Build history of the part. All positions in model axes, mm. A direction names the side the tool comes from. Round coordinates to 2 decimals unless told otherwise and drop trailing zeros. Write each loop counter-clockwise with the first axis right and the second up, starting at its lowest first coordinate (ties: lowest second). Pieces come first, ordered by that corner, then holes. Notation, with made-up numbers: (-9, 50.25) - (33, 50.25) arc R22 cw to (33, 79.25) - close; hole circle Ø3 at (37, 3.5). An arc over 180 degrees is marked (long way). Answer as a JSON object with one key per item and string values. Group by question number.
Item 1: Probe line 1 (Y direction, x = 14, z = -1.75); line 2 (Y direction, x = 37, z = -0.25). List the from-to ranges inside material, lowest first. Write a range as from..to.
Item 2: Slice it at A-A, the plane z = 0. List the corners of the cut face in (x, y) (3 decimals), then the cut area to 3 significant figures.
Item 3: Slice it at B-B, the plane y = 0. List the corners of the cut face in (x, z) (3 decimals).
Item 4: Two-plate mould, pull along Y, no slides. Class faces 3 (the cylindrical face through (24.46, -2.861, 9.085)), 4 (the flat face through (50.8, 0, 0)), 5 (the flat face through (3, 1.702, 0)): +Y half, -Y half, draft (parallel to the pull), parting line (faces both ways), or undercut.
Item 5: Slice it at D-D, the plane x = 40.5. List the corners of the cut face in (y, z) (3 decimals), then the cut area to 3 significant figures.
Item 6: Which spindle directions (+Z, -Z, +X, -X, +Y, -Y) get a long thin tool onto all of the face, cutting with end or side? Do faces 1 (the flat face through (4.902, 0, 0)), 2 (the conical face through (50.56, 5.28, 2.75)). Say none if no direction does.
Item 7: Flat gauge pins, fed straight in: pin 1 (2 mm diameter, centred on x = 37, y = 6, fed in from +Z); pin 2 (5.5 mm diameter, centred on x = 1.5, z = 2.5, fed in from +Y) (3 decimals); pin 3 (10 mm diameter, centred on x = 26, y = 6, fed in from +Z); pin 4 (1.5 mm diameter, centred on x = 33.5, y = -6.5, fed in from +Z). Where does each tip first touch, or does it go through?
Item 8: Slice it at C-C, the plane x = 3.5. List the corners of the cut face in (y, z) (3 decimals), then the cut area to 3 significant figures.
from build123d import *

# Parameters (mm, degrees)
SKETCH2_W  = 19.05
SKETCH2_H  = 3.4036
SLOT_DEPTH = 4.9022


with BuildPart() as part:
    # BodySke → BaseBody (revolve)
    with BuildSketch(Plane.XY, mode=Mode.PRIVATE) as basebody_sk:
        with BuildLine():
            Line((50.8, 0), (50.8, 5.715))
            Line((50.8, 5.715), (46.99, 9.525))
            Line((46.99, 9.525), (2.552216058, 9.525))
            ThreePointArc((2.552216058, 9.525), (0.649113009, 4.930502809), (0, 0))
            Line((0, 0), (50.8, 0))
        make_face()
    revolve(basebody_sk.sketch.rotate(Axis((-12.7, 0, 0), (1, 0, 0)), 90), axis=Axis((-12.7, 0, 0), (1, 0, 0)))

    # Sketch2 → Slot (cut)
    with BuildSketch(Plane(origin=(0, 0, 0), x_dir=(0, 0, -1), z_dir=(1, 0, 0))):
        Rectangle(SKETCH2_W, SKETCH2_H)
    extrude(amount=SLOT_DEPTH, mode=Mode.SUBTRACT)


solid = part.part
Geometry says:
{
 "1": {"line 1": "y = -9.36..9.36", "line 2": "y = -9.52..9.52"},
 "2": {"outline": "(0.076, -1.702) arc R19.05 ccw to (2.552, -9.525) - (46.99, -9.525) - (50.8, -5.715) - (50.8, 5.715) - (46.99, 9.525) - (2.552, 9.525) arc R19.05 ccw to (0.076, 1.702) - (4.902, 1.702) - (4.902, -1.702) - close", "area": "921 mm^2"},
 "3": {"outline": "(4.902, -9.525) - (46.99, -9.525) - (50.8, -5.715) - (50.8, 5.715) - (46.99, 9.525) - (4.902, 9.525) - close"},
 "4": {"face 3": "parting line", "face 4": "draft", "face 5": "undercut"},
 "5": {"outline": "circle Ø19.05 at (0, 0)", "area": "285 mm^2"},
 "6": {"face 1": "+Z, -Z, -X", "face 2": "+X"},
 "7": {"pin 1": "stops at z = 8.11", "pin 2": "stops at y = 9.525", "pin 3": "stops at z = 9.47", "pin 4": "stops at z = 7.59"},
 "8": {"outline": "(-1.702, -9.372) - (-1.702, 9.372) arc R9.525 ccw to start; (1.702, -9.372) arc R9.525 ccw to (1.702, 9.372) - close", "area": "221 mm^2"}
}
